Source: CAD feature listing. Evaluate the final solid. Frame: model axes, mm. Face numbers are marked on the shaded views. Round coordinates to 2 decimals unless told otherwise and drop trailing zeros. Loops run counter-clockwise (first coordinate to the right, second up) from the corner with the lowest first, then second, coordinate; pieces in that order, holes last.
Item 1: Pull-direction query (Y, two-part tool) for the marked faces 1, 2, 3 and 4; classes: released by +Y, released by -Y, zero draft, split by the parting line, or undercut.
Item 2: Section query B-B on x = 0. Return loops of the section in (y, z), then the cut area to 3 significant figures.
Item 3: First-contact query: P1, Ø2, axis at x = -28.5, y = 18, coming from the -Z side. Flat tip, straight axial feed; report the tip coordinate or a pass-through.
Item 4: Section query A-A on y = -16. Return loops of the section in (x, z).
Item 5: Section query C-C on z = 31. Return loops of the section in (x, y).
Item 6: Ray query, L1, parallel to Y at x = -50, z = 29.5; L2, parallel to X at y = 12.5, z = 18; L3, parallel to X at y = -14.5, z = 6.5. Return the intervals inside material, ascending.
Item 7: Section query D-D on y = 0. Return loops of the section in (x, z).
```python
from build123d import *

# Parameters (mm, degrees)
SKETCH_W        = 200
SKETCH_H        = 75
SKETCH_R        = 20
PAD_DEPTH       = 45
CHAMFER_SIZE    = 3
CHAMFER001_SIZE = 3


with BuildPart() as part:
    # Sketch → Pad (new body)
    with BuildSketch(Plane.XY):
        Rectangle(SKETCH_W, SKETCH_H)
        Circle(SKETCH_R, mode=Mode.SUBTRACT)
        with Locations((-50, 0)):
            Circle(SKETCH_R, mode=Mode.SUBTRACT)
        with Locations((50, 0)):
            Circle(SKETCH_R, mode=Mode.SUBTRACT)
    extrude(amount=PAD_DEPTH)

    # Chamfer
    chamfer_edges = [part.edges().sort_by_distance(p)[0] for p in [
        (100, 0, 45),
        (0, 37.5, 45),
        (-100, 0, 45),
        (0, -37.5, 45),
    ]]
    chamfer(chamfer_edges, length=CHAMFER_SIZE)

    # Chamfer001
    chamfer001_edges = [part.edges().sort_by_distance(p)[0] for p in [
        (100, 37.5, 21),
        (100, -37.5, 21),
        (-100, -37.5, 21),
        (-100, 37.5, 21),
    ]]
    chamfer(chamfer001_edges, length=CHAMFER001_SIZE)


solid = part.part
```
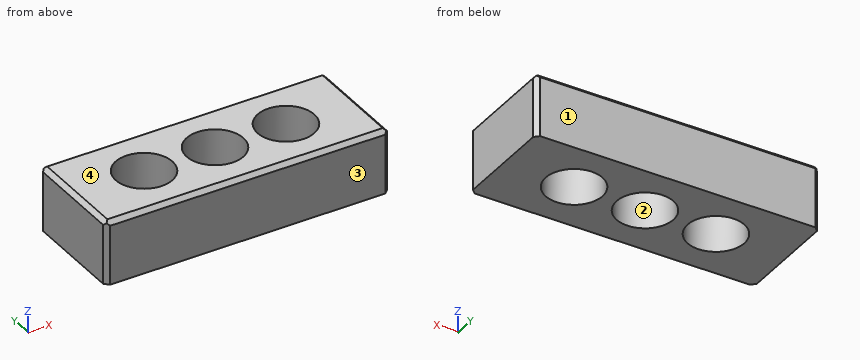
Data:
1. face 1: released by +Y
1. face 2: undercut
1. face 3: released by -Y
1. face 4: zero draft
2. outline: (-37.5, 0) - (-20, 0) - (-20, 45) - (-34.5, 45) - (-37.5, 42) - close; (20, 0) - (37.5, 0) - (37.5, 42) - (34.5, 45) - (20, 45) - close
2. area: 1,570 mm2
3. P1: stops at z = 0
4. outline: (-100, 0) - (-62, 0) - (-62, 45) - (-97, 45) - (-100, 42) - close; (-38, 0) - (-12, 0) - (-12, 45) - (-38, 45) - close; (12, 0) - (38, 0) - (38, 45) - (12, 45) - close; (62, 0) - (100, 0) - (100, 42) - (97, 45) - (62, 45) - close
5. outline: (-100, -34.5) - (-97, -37.5) - (97, -37.5) - (100, -34.5) - (100, 34.5) - (97, 37.5) - (-97, 37.5) - (-100, 34.5) - close; hole circle Ø40 at (-50, 0); hole circle Ø40 at (0, 0); hole circle Ø40 at (50, 0)
6. L1: y = -37.5 to -20, 20 to 37.5
6. L2: x = -100 to -65.61, -34.39 to -15.61, 15.61 to 34.39, 65.61 to 100
6. L3: x = -100 to -63.77, -36.23 to -13.77, 13.77 to 36.23, 63.77 to 100
7. outline: (-100, 0) - (-70, 0) - (-70, 45) - (-97, 45) - (-100, 42) - close; (-30, 0) - (-20, 0) - (-20, 45) - (-30, 45) - close; (20, 0) - (30, 0) - (30, 45) - (20, 45) - close; (70, 0) - (100, 0) - (100, 42) - (97, 45) - (70, 45) - close
